Design review of the part built by this model. Coordinates are the model's own, in mm. Face numbers are marked on the shaded views. Coordinates: 2 decimals unless noted, no trailing zeros. Loops run counter-clockwise (first coordinate to the right, second up) from the corner with the lowest first, then second, coordinate; pieces in that order, holes last. Notation, with made-up numbers: (-21, 89.25) - (1, 89.25) arc R9 ccw to (1, 96.25) - close; hole circle Ø3 at (28.25, 24.5). An arc over 180 degrees is marked (long way). One line per question, with ' | ' between items.
from build123d import *


with BuildPart() as f1:
    # F0 (on Front) → F1 (revolve)
    with BuildSketch(Plane.XZ):
        with BuildLine():
            Line((-26.951872, -47.867652), (-14.87968, -47.867652))
            Line((-14.87968, -47.867652), (-14.87968, -11.089573))
            Line((-14.87968, -11.089573), (0, -11.089573))
            Line((0, -11.089573), (0, 5.749613))
            add(Edge.make_bspline(
                [(0, 47.311883), (-11.906475, 47.311883), (-11.906475, 26.530748), (-11.906475, 5.749613), (0, 5.749613)],
                knots=[3.141593, 3.141593, 3.141593, 4.712389, 4.712389, 6.283185, 6.283185, 6.283185], degree=2, weights=[1, 0.707107, 1, 0.707107, 1]))
            Line((0, 47.311883), (0, 52.858687))
            Line((0, 52.858687), (-16.830357, 52.858687))
            ThreePointArc((-16.830357, 52.858687), (-18.463521, 52.375187), (-19.570262, 51.080536))
            Line((-19.570262, 51.080536), (-36.778077, 12.493316))
            Line((-36.778077, 12.493316), (-36.778077, 0))
            Line((-36.778077, 0), (-26.951872, 0))
            Line((-26.951872, 0), (-26.951872, -47.867652))
        make_face()
    revolve(axis=Axis((0, 0, 20.884557), (0, 0, -1)))


solid = f1.part
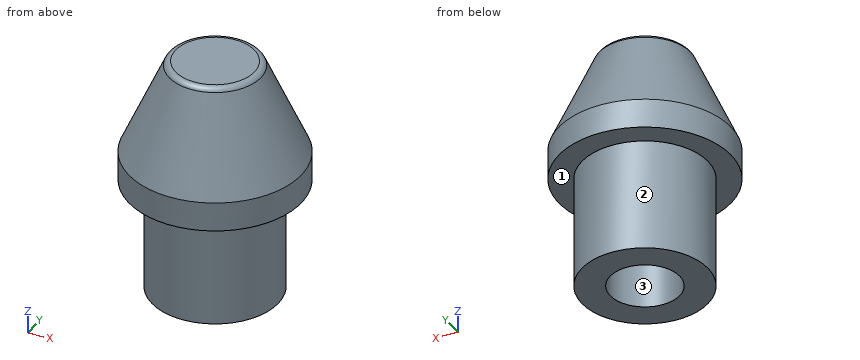
Q1. For pin 1 (15 mm diameter, centred on x = 2.5, y = -1.5, fed in from -Z); pin 2 (1 mm diameter, centred on y = 4, z = 2, fed in from +X); pin 3 (1.5 mm diameter, centred on x = -27, z = 22, fed in from -Y), all flat-tipped, find the tip position at first contact; note any pin that passes through.
Returned:
pin 1: stops at z = -11.09 | pin 2: stops at x = 36.61 | pin 3: stops at y = -19.37
Q2. To check wall thickness, follow line 1 along Y through (x, z) = (0, -28.5); line 2 along Z through (x, y) = (-3.5, 13); line 3 along Y through (x, z) = (-5, 42.5). State the ranges of each line that lie inside material, in increasing order.
Returned:
line 1: y = -26.95 to -14.88, 14.88 to 26.95 | line 2: z = -11.09 to 52.86 | line 3: y = -22.86 to -5.75, 5.75 to 22.86
Q3. Draft analysis for pull direction X (two halves, no side actions). For the marked faces 1, 2 and 3, state which applies: +X half, -X half, draft (parallel to the pull), parting line (faces both ways), or undercut.
Returned:
face 1: draft | face 2: parting line | face 3: undercut
Q4. Take a section at A-A (z = -28). Give the boundary of the cut face in (x, y), plus the area to 3 significant figures.
Returned:
outline: circle Ø53.9 at (0, 0); hole circle Ø29.76 at (0, 0) | area: 1,590 mm²
Q5. Take a section at B-B (z = -8.5). Give the boundary of the cut face in (x, y), plus the area to 3 significant figures.
Returned:
outline: circle Ø53.9 at (0, 0) | area: 2,280 mm²
